from build123d import *

# Parameters (mm, degrees)
F1_DEPTH = 10
F2_W     = 6
F2_H     = 14.9
F3_DEPTH = 2
F5_R     = 0.5
F7_D     = 3


with BuildPart() as f1:
    # F0 (on Front) → F1 (new body)
    with BuildSketch(Plane.XZ):
        Polygon((3.6, 0), (0, 0), (0, -3), (12, -3), (12, 11.9), (8.4125, 11.9), (3.6, 5), align=None)
    extrude(amount=-F1_DEPTH)

    # F2 (on face) → F3 (cut)
    with BuildSketch(Plane.YZ.offset(12)):
        with Locations((5, 4.45)):
            Rectangle(F2_W, F2_H)
    extrude(amount=-F3_DEPTH, mode=Mode.SUBTRACT)

    # F4: F1 across plane


with BuildPart() as f1_1:
    add(f1.part)
    add(f1.part.mirror(Plane.YZ))

    # F5
    f5_edges = [f1_1.edges().sort_by_distance(p)[0] for p in [
        (-8.4125, 5, 11.9),
        (-12, 1, 11.9),
        (-12, 9, 11.9),
        (-3.6, 5, 5),
        (-3.6, 5, 0),
        (3.6, 5, 0),
        (3.6, 5, 5),
        (8.4125, 5, 11.9),
        (12, 9, 11.9),
        (12, 1, 11.9),
        (12, 9, -3),
        (12, 1, -3),
        (-12, 1, -3),
        (-12, 9, -3),
        (10, 8, 4.45),
        (10, 2, 4.45),
        (-10, 2, 4.45),
        (-10, 8, 4.45),
    ]]
    fillet(f5_edges, radius=F5_R)

    # F7 (through all)
    with Locations(Plane(origin=(0, 0, -3), x_dir=(1, 0, 0), z_dir=(0, 0, -1))):
        with Locations((0, -5)):
            Hole(F7_D / 2)


solid = f1_1.part
Part model, mm, in its own coordinate system. A direction names the side the tool comes from. Coordinates: 2 decimals unless noted, no trailing zeros. Write each loop counter-clockwise with the first axis right and the second up, starting at its lowest first coordinate (ties: lowest second). Pieces come first, ordered by that corner, then holes. Notation, with made-up numbers: M 35.25,48 L 82.25,48 A29 cw 82.25,80 Z; hole C 61,70 d3. An arc over 180 degrees is marked long. Return JSON: item names as keys, results as strings.
1. Flat gauge pins, fed straight in: pin 1 Ø1.5 at (y, z) = (4.5, 6.5) entering from +X; pin 2 Ø2.5 at (y, z) = (4, 7.5) entering from -X. Where does each tip first touch, or does it go through?
Determined:
{"pin 1": "x = 10", "pin 2": "x = -10"}
2. Pull direction X, two halves, no side cores. Call faces 1 (the face through (6.009, 4.93, 8.453)), 2 (the face through (11, 8, 4)), 3 (the face through (10, 5, 5)): pulls with the +X half, pulls with the -X half, needs draft (parallel to the pull), parting line crosses it, or undercut.
Determined:
{"face 1": "undercut", "face 2": "needs draft", "face 3": "pulls with the +X half"}
3. Saw through at B-B, the plane y = 5. Write the cut outline in (x, z), then the cut area to 3 significant figures.
Determined:
{"outline": "M -10,-3 L -1.5,-3 L -1.5,0 L -3.1,0 A0.5 cw -3.6,0.5 L -3.6,4.84 A0.5 ccw -3.69,5.13 L -8.26,11.69 A0.5 ccw -8.67,11.9 L -10,11.9 Z; M 1.5,-3 L 10,-3 L 10,11.9 L 8.67,11.9 A0.5 ccw 8.26,11.69 L 3.69,5.13 A0.5 ccw 3.6,4.84 L 3.6,0.5 A0.5 cw 3.1,0 L 1.5,0 Z", "area": "170 mm²"}
4. 3-axis set-ups, long thin cutter, end or side, ignore diameter. For faces 4 (the face through (-11, 2, 4)), 5 (the face through (0, 3, -3)), 6 (the face through (3.6, 5, 3)): which of +Z, -Z, +X, -X, +Y, -Y reach the whole face in a straight line?
Determined:
{"face 4": "+Z, -Z, -X", "face 5": "-Z, +X, -X, +Y, -Y", "face 6": "+Z, +Y, -Y"}
5. Probe L1, parallel to Y at x = 0, z = -1.35; L2, parallel to X at y = 5, z = -2.2; L3, parallel to X at y = 9.75, z = 2.25. List the from-to ranges inside material, lowest first.
Determined:
{"L1": "0 to 3.5, 6.5 to 10", "L2": "-10 to -1.5, 1.5 to 10", "L3": "-12 to -3.6, 3.6 to 12"}
6. Saw through at C-C, the plane z = 11. Write the cut outline in (x, y).
Determined:
{"outline": "M -12,0 L -7.78,0 L -7.78,10 L -12,10 L -12,8 L -10.5,8 A0.5 cw -10,7.5 L -10,2.5 A0.5 cw -10.5,2 L -12,2 Z; M 7.78,0 L 12,0 L 12,2 L 10.5,2 A0.5 cw 10,2.5 L 10,7.5 A0.5 cw 10.5,8 L 12,8 L 12,10 L 7.78,10 Z"}
7. Saw through at D-D, the plane y = 3. Write the cut outline in (x, z).
Determined:
{"outline": "M -10,-3 L 10,-3 L 10,11.9 L 8.67,11.9 A0.5 ccw 8.26,11.69 L 3.69,5.13 A0.5 ccw 3.6,4.84 L 3.6,0.5 A0.5 cw 3.1,0 L -3.1,0 A0.5 cw -3.6,0.5 L -3.6,4.84 A0.5 ccw -3.69,5.13 L -8.26,11.69 A0.5 ccw -8.67,11.9 L -10,11.9 Z"}
8. Saw through at A-A, the plane x = 0. Write the cut outline in (y, z).
Determined:
{"outline": "M 0,-3 L 3.5,-3 L 3.5,0 L 0,0 Z; M 6.5,-3 L 10,-3 L 10,0 L 6.5,0 Z"}
